Verification items for the finished model (mm, model axes). Face numbers are marked on the shaded views. A direction names the side the tool comes from. Coordinates: 2 decimals unless noted, no trailing zeros. Loops run counter-clockwise (first coordinate to the right, second up) from the corner with the lowest first, then second, coordinate; pieces in that order, holes last. Notation, with made-up numbers: (59.5, 22) -> (81.5, 22) arc R6 cw to (81.5, 28) -> close; hole circle Ø9 at (4.5, 38.25). An arc over 180 degrees is marked (long way). Answer as a JSON object with one key per item and string values. Group by question number.
Q1. Cross-section at A-A on z = -7. Record the boundary of the cut face in (x, y), and give its area (3 significant figures).
Q2. Cross-section at B-B on y = 18.25. Record the boundary of the cut face in (x, z).
Q3. Gauge pin test, flat ends, axial feed: pin 1 Ø5 at (y, z) = (2.5, -4) entering from +X; pin 2 Ø1.5 at (y, z) = (3.5, -32.5) entering from -X. Record the tip position at first contact, or that the pin passes through.
Q4. Release check for a two-part mould opening along X. For the marked faces 1, 2 and 3 record: released by +X, released by -X, zero draft, split by the parting line, or undercut.
Q5. Scan line: L1, parallel to X at y = 8.25, z = -42.5. Record every from-to range of solid material in increasing order.
Q6. Set-up check for the marked faces 4 and 5: record each of +Z, -Z, +X, -X, +Y, -Y from which the full face is reachable in a straight line by a thin tool's end or side.
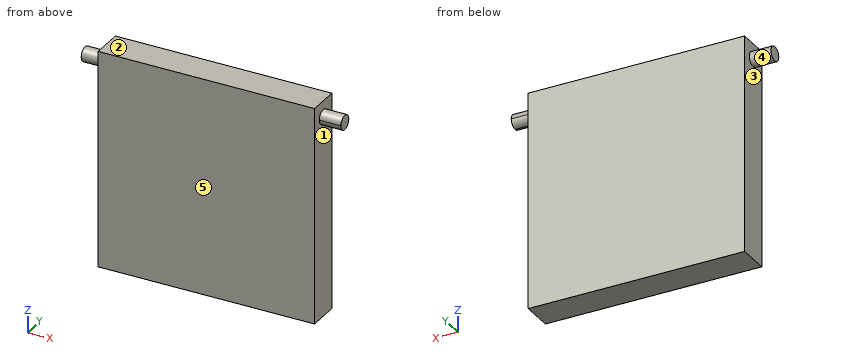
```python
from build123d import *

# Parameters (mm, degrees)
ESQUISSE1_W        = 150
ESQUISSE1_H        = 150
BOSS_EXTRU_1_DEPTH = 22
BOSS_EXTRU_2_DEPTH = 15
BOSS_EXTRU_3_START = 15
ESQUISSE6_R        = 5
BOSS_EXTRU_3_DEPTH = 15


with BuildPart() as part:
    # Esquisse1 → Boss.-Extru.1 (new body)
    with BuildSketch(Plane(origin=(0, 0, 0), x_dir=(1, 0, 0), z_dir=(0, 1, 0))):
        Rectangle(ESQUISSE1_W, ESQUISSE1_H)
    extrude(amount=BOSS_EXTRU_1_DEPTH)

    # Esquisse2 → Boss.-Extru.2 (add)
    with BuildSketch(Plane(origin=(75, 0, 0), x_dir=(0, 0, -1), z_dir=(1, 0, 0))):
        with BuildLine():
            ThreePointArc((-64, 16), (-69, 11), (-64, 6))
            Line((-64, 6), (-64, 16))
        make_face()
        with BuildLine():
            Line((-64, 16), (-64, 6))
            ThreePointArc((-64, 6), (-60.464466094, 7.464466094), (-59, 11))
            ThreePointArc((-59, 11), (-60.464466094, 14.535533906), (-64, 16))
        make_face()
    extrude(amount=BOSS_EXTRU_2_DEPTH)

    # Esquisse6 → Boss.-Extru.3 (add)
    with BuildSketch(Plane.ZY.offset(75).offset(BOSS_EXTRU_3_START)):
        with Locations((64, 11)):
            Circle(ESQUISSE6_R)
    extrude(amount=-BOSS_EXTRU_3_DEPTH)


solid = part.part
```
Computed values:
{
 "1": {"outline": "(-75, 0) -> (75, 0) -> (75, 22) -> (-75, 22) -> close", "area": "3,300 mm²"},
 "2": {"outline": "(-75, -75) -> (75, -75) -> (75, 75) -> (-75, 75) -> close"},
 "3": {"pin 1": "stops at x = 75", "pin 2": "stops at x = -75"},
 "4": {"face 1": "released by +X", "face 2": "zero draft", "face 3": "released by -X"},
 "5": {"L1": "x = -75 to 75"},
 "6": {"face 4": "-X", "face 5": "+Z, -Z, +X, -X, -Y"}
}
